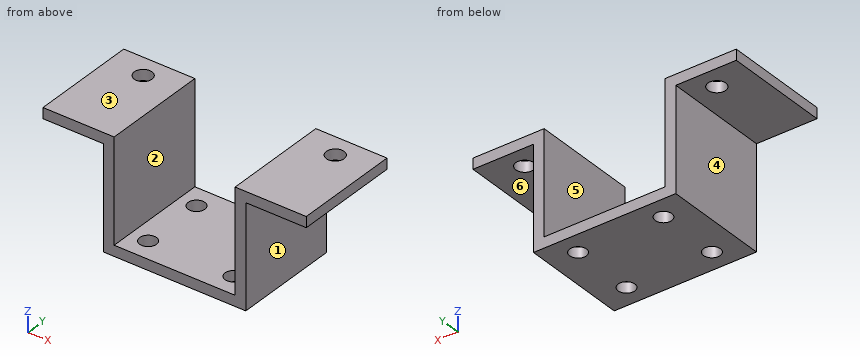
```python
from build123d import *

# Parameters (mm, degrees)
SKETCH1_W           = 3
SKETCH1_H           = 3
SKETCH1_W_2         = 17
BOSS_EXTRUDE1_DEPTH = 30
SKETCH2_R           = 2.5
CUT_EXTRUDE1_DEPTH  = 30
SKETCH3_R           = 2.35
CUT_EXTRUDE2_DEPTH  = 30


with BuildPart() as part:
    # Sketch1 → Boss-Extrude1 (new body)
    with BuildSketch(Plane(origin=(0, 0, 0), x_dir=(1, 0, 0), z_dir=(0, 1, 0))):
        Polygon((-17, 29), (0, 29), (17, 29), (17, 3), (20, 3), (20, 32), (-20, 32), (-20, 3), (-17, 3), align=None)
        with Locations((-18.5, 1.5)):
            Rectangle(SKETCH1_W, SKETCH1_H)
        with Locations((-28.5, 1.5)):
            Rectangle(SKETCH1_W_2, SKETCH1_H)
        with Locations((18.5, 1.5)):
            Rectangle(SKETCH1_W, SKETCH1_H)
        with Locations((28.5, 1.5)):
            Rectangle(SKETCH1_W_2, SKETCH1_H)
    extrude(amount=BOSS_EXTRUDE1_DEPTH)

    # Sketch2 → Cut-Extrude1 (cut)
    with BuildSketch(Plane.XY):
        with Locations((-27, 24)):
            Circle(SKETCH2_R)
        with Locations((27, 24)):
            Circle(SKETCH2_R)
    extrude(amount=-CUT_EXTRUDE1_DEPTH, mode=Mode.SUBTRACT)

    # Sketch3 → Cut-Extrude2 (cut)
    with BuildSketch(Plane(origin=(0, 0, -32), x_dir=(-1, 0, 0), z_dir=(0, 0, -1))):
        with Locations((-12, 6)):
            Circle(SKETCH3_R)
        with Locations((12, 6)):
            Circle(SKETCH3_R)
        with Locations((12, 24)):
            Circle(SKETCH3_R)
        with Locations((-12, 24)):
            Circle(SKETCH3_R)
    extrude(amount=-CUT_EXTRUDE2_DEPTH, mode=Mode.SUBTRACT)


solid = part.part
```
The listing builds one solid part. Answer for the finished solid, in the listing's coordinates (mm). Face numbers are marked on the shaded views. A direction names the side the tool comes from. Give positions to 0.01 mm unless a question says otherwise; leave off trailing zeros. Loops run counter-clockwise (first coordinate to the right, second up) from the corner with the lowest first, then second, coordinate; pieces in that order, holes last. Notation, with made-up numbers: (-10, 44) - (-6, 44) arc R13 ccw to (-6, 50) - close; hole circle Ø5 at (8.5, 36.25). An arc over 180 degrees is marked (long way). Return JSON: item names as keys, results as strings. Group by question number.
1. Which of the six approach directions +Z, -Z, +X, -X, +Y, -Y give full straight-line access (tool end or side, diameter ignored) to the marked faces 4, 5 and 6?
2. Find section C-C (y = 24). Write down the section's boundary in (x, z), then the cut area to 3 significant figures.
3. Given pin 1 Ø10 at (y, z) = (21, -8.5) entering from -X; pin 2 Ø13.5 at (x, y) = (-27, 8.5) entering from -Z; pin 3 Ø2 at (x, y) = (-29.5, 21) entering from +Z; pin 4 Ø1 at (x, y) = (5, 6) entering from +Z, each flat-ended and moving along its own axis, determine where each tip first touches the part or whether it passes through.
4. Determine the mould class of the marked faces 1, 2 and 3 for opening direction X: pulls with the +X half, pulls with the -X half, needs draft (parallel to the pull), parting line crosses it, or undercut.
5. Find section A-A (x = -27). Write down the section's boundary in (y, z).
6. Find section D-D (x = -12). Write down the section's boundary in (y, z).
7. Find section B-B (z = -15.5). Write down the section's boundary in (x, y), then the cut area to 3 significant figures.
8. Straight lines are drawn through the part: line 1 (X direction, y = 18, z = -7); line 2 (Y direction, x = -12, z = -29.95); line 3 (X direction, y = 17.75, z = -2). For each, find the intervals that lie inside material, in ascending order. Write a range as [from, to].
Verdict:
{
 "1": {"face 4": "-Z, -X, +Y, -Y", "face 5": "+Z, +Y, -Y", "face 6": "-Z, +X, +Y, -Y"},
 "2": {"outline": "(-37, -3) - (-29.5, -3) - (-29.5, 0) - (-37, 0) - close; (-24.5, -3) - (-20, -3) - (-20, -32) - (-14.35, -32) - (-14.35, -29) - (-17, -29) - (-17, 0) - (-24.5, 0) - close; (-9.65, -32) - (9.65, -32) - (9.65, -29) - (-9.65, -29) - close; (14.35, -32) - (20, -32) - (20, -3) - (24.5, -3) - (24.5, 0) - (17, 0) - (17, -29) - (14.35, -29) - close; (29.5, -3) - (37, -3) - (37, 0) - (29.5, 0) - close", "area": "338 mm^2"},
 "3": {"pin 1": "stops at x = -20", "pin 2": "stops at z = -3", "pin 3": "stops at z = 0", "pin 4": "stops at z = -29"},
 "4": {"face 1": "pulls with the +X half", "face 2": "undercut", "face 3": "needs draft"},
 "5": {"outline": "(0, -3) - (21.5, -3) - (21.5, 0) - (0, 0) - close; (26.5, -3) - (30, -3) - (30, 0) - (26.5, 0) - close"},
 "6": {"outline": "(0, -32) - (3.65, -32) - (3.65, -29) - (0, -29) - close; (8.35, -32) - (21.65, -32) - (21.65, -29) - (8.35, -29) - close; (26.35, -32) - (30, -32) - (30, -29) - (26.35, -29) - close"},
 "7": {"outline": "(-20, 0) - (-17, 0) - (-17, 30) - (-20, 30) - close; (17, 0) - (20, 0) - (20, 30) - (17, 30) - close", "area": "180 mm^2"},
 "8": {"line 1": "x = [-20, -17], [17, 20]", "line 2": "y = [0, 3.65], [8.35, 21.65], [26.35, 30]", "line 3": "x = [-37, -17], [17, 37]"}
}
